Build history of the part. All positions in model axes, mm. Face numbers are marked on the shaded views. A direction names the side the tool comes from. Give positions to 0.01 mm unless a question says otherwise; leave off trailing zeros. Write each loop counter-clockwise with the first axis right and the second up, starting at its lowest first coordinate (ties: lowest second). Pieces come first, ordered by that corner, then holes.
from build123d import *

# Parameters (mm, degrees)
ESQUISSE1_W             = 13
ESQUISSE1_H             = 18
BOSS_EXTRU_1_DEPTH      = 12
ENL_V_MAT_EXTRU_1_DEPTH = 12


with BuildPart() as part:
    # Esquisse1 → Boss.-Extru.1 (new body)
    with BuildSketch(Plane.XY):
        Rectangle(ESQUISSE1_W, ESQUISSE1_H)
    extrude(amount=BOSS_EXTRU_1_DEPTH)

    # Esquisse2 → Enlèv. mat.-Extru.1 (cut)
    with BuildSketch(Plane.XZ.offset(9)):
        Polygon((-5, 10), (-3, 10), (-3, 12), (3, 12), (3, 10), (5, 10), (5, 2), (3, 2), (3, 0), (-3, 0), (-3, 2), (-5, 2), align=None)
    extrude(amount=-ENL_V_MAT_EXTRU_1_DEPTH, mode=Mode.SUBTRACT)


solid = part.part
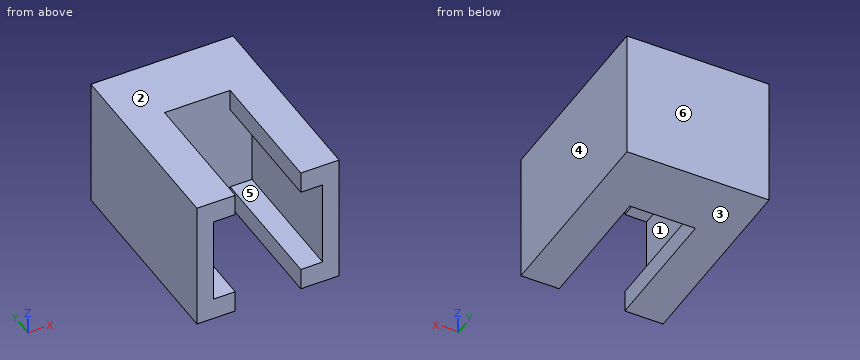
1. Saw through at D-D on x = 2. Give the cut face in (y, z), plus the area to 3 significant figures.
2. Drill centre lines: line 1 along X through (y, z) = (-2.75, 3); line 2 along X through (y, z) = (-4.5, 10.75); line 3 along Z through (x, y) = (4, -0.25). Where is each one in solid material? Low to high.
3. Saw through at B-B on z = 7. Give the cut face in (x, y).
4. Saw through at C-C on x = 4. Give the cut face in (y, z), plus the area to 3 significant figures.
5. Mould opens along Z. For the marked faces 1, 2, 3 and 4 say: pulls with the +Z half, pulls with the -Z half, needs draft (parallel to the pull), parting line crosses it, or undercut.
6. Saw through at A-A on y = 0. Give the cut face in (x, z).
7. 3-axis set-ups, long thin cutter, end or side, ignore diameter. For the marked faces 5 and 6: which of +Z, -Z, +X, -X, +Y, -Y reach the whole face in a straight line?
Outcome:
1. outline: (3, 0) - (9, 0) - (9, 12) - (3, 12) - close
1. area: 72.0 mm2
2. line 1: x = -6.5 to -5, 5 to 6.5
2. line 2: x = -6.5 to -3, 3 to 6.5
2. line 3: z = 0 to 2, 10 to 12
3. outline: (-6.5, -9) - (-5, -9) - (-5, 3) - (5, 3) - (5, -9) - (6.5, -9) - (6.5, 9) - (-6.5, 9) - close
4. outline: (-9, 0) - (9, 0) - (9, 12) - (-9, 12) - (-9, 10) - (3, 10) - (3, 2) - (-9, 2) - close
4. area: 120 mm2
5. face 1: undercut
5. face 2: pulls with the +Z half
5. face 3: pulls with the -Z half
5. face 4: needs draft
6. outline: (-6.5, 0) - (-3, 0) - (-3, 2) - (-5, 2) - (-5, 10) - (-3, 10) - (-3, 12) - (-6.5, 12) - close; (3, 0) - (6.5, 0) - (6.5, 12) - (3, 12) - (3, 10) - (5, 10) - (5, 2) - (3, 2) - close
7. face 5: -Y
7. face 6: +Z, -Z, +X, -X, +Y
